from build123d import *

# Parameters (mm, degrees)
BOSS_EXTRUDE1_DEPTH = 1.27
FILLET1_R           = 1.143


with BuildPart() as part:
    # Sketch1 → Boss-Extrude1 (new body, symmetric)
    with BuildSketch(Plane(origin=(0, 0, 0), x_dir=(1, 0, 0), z_dir=(0, 1, 0))):
        Polygon((0, 0), (81.28, 0), (81.28, -58.049008178), (3.729896149, -53.34), align=None)
    extrude(amount=BOSS_EXTRUDE1_DEPTH, both=True)

    # Fillet1
    fillet1_edges = [part.edges().sort_by_distance(p)[0] for p in [
        (42.504948075, -1.27, 55.694504089),
        (42.504948075, 1.27, 55.694504089),
    ]]
    fillet(fillet1_edges, radius=FILLET1_R)


solid = part.part
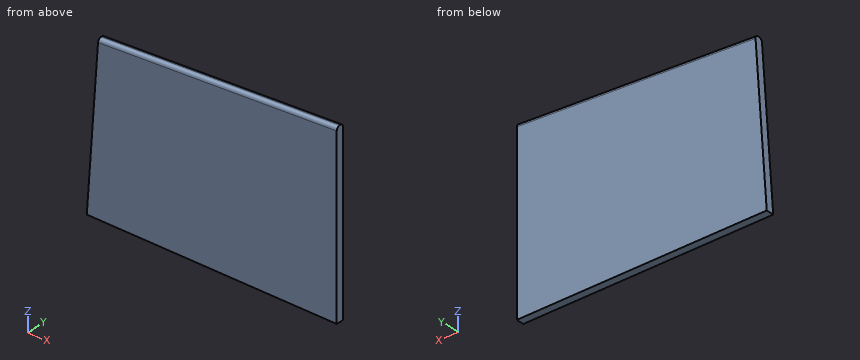
The listing builds one solid part. Answer for the finished solid, in the listing's coordinates (mm). Give positions to 0.01 mm unless a question says otherwise; leave off trailing zeros. Loops run counter-clockwise (first coordinate to the right, second up) from the corner with the lowest first, then second, coordinate; pieces in that order, holes last.
Item 1: Find the intervals of material crossed by line 1 along Z through (x, y) = (34.5, 0.85); line 2 along Z through (x, y) = (29, -0.65); line 3 along X through (y, z) = (-0.45, 53), in increasing order.
Derived:
line 1: z = 0 to 54.95
line 2: z = 0 to 54.75
line 3: x = 3.71 to 81.28
Item 2: A cutting plane is placed at B-B (y = -0.75). Give the vertices of the cut face in (x, z).
Derived:
outline: (0, 0) - (81.28, 0) - (81.28, 57.86) - (3.72, 53.15) - close
Item 3: A cutting plane is placed at A-A (z = 18). Give the vertices of the cut face in (x, y), then the cut area to 3 significant figures.
Derived:
outline: (1.26, -1.27) - (81.28, -1.27) - (81.28, 1.27) - (1.26, 1.27) - close
area: 203 mm2
